```python
from build123d import *
from OCP.BRepFilletAPI import BRepFilletAPI_MakeChamfer

# Parameters (mm, degrees)
SKETCH1_R           = 2
BOSS_EXTRUDE1_DEPTH = 47
BOSS_EXTRUDE2_DEPTH = 4
FILLET1_R           = 0.2
CUT_EXTRUDE2_DEPTH  = 1
CUT_EXTRUDE2_DRAFT  = -12
CHAMFER1_SIZE       = 0.2
CHAMFER1_SIZE_2     = 0.259660706


with BuildPart() as part:
    # Sketch1 → Boss-Extrude1 (new body)
    with BuildSketch(Plane(origin=(0, 0, 0), x_dir=(1, 0, 0), z_dir=(0, 1, 0))):
        with Locations(Location((0, 0, 0), (0, 0, 270))):
            Circle(SKETCH1_R)
    extrude(amount=-BOSS_EXTRUDE1_DEPTH)

    # Sketch2 → Boss-Extrude2 (add)
    with BuildSketch(Plane(origin=(0, 0, 0), x_dir=(1, 0, 0), z_dir=(0, 1, 0))):
        Polygon((0, 5.196152423), (-4.5, 2.598076211), (-4.5, -2.598076211), (0, -5.196152423), (4.5, -2.598076211), (4.5, 2.598076211), align=None)
    extrude(amount=BOSS_EXTRUDE2_DEPTH)

    # Fillet1
    fillet1_edges = [part.edges().sort_by_distance(p)[0] for p in [
        (2.25, 0, -3.897114317),
        (4.5, 2, -2.598076211),
        (-2.25, 0, -3.897114317),
        (0, 2, -5.196152423),
        (-4.5, 0, 0),
        (-4.5, 2, -2.598076211),
        (-2.25, 0, 3.897114317),
        (-4.5, 2, 2.598076211),
        (2.25, 0, 3.897114317),
        (0, 2, 5.196152423),
        (4.5, 0, 0),
        (4.5, 2, 2.598076211),
        (2.25, 4, -3.897114317),
        (-2.25, 4, -3.897114317),
        (-4.5, 4, 0),
        (-2.25, 4, 3.897114317),
        (2.25, 4, 3.897114317),
        (4.5, 4, 0),
    ]]
    fillet(fillet1_edges, radius=FILLET1_R)


with BuildPart() as cut_extrude2_tool:
    # Sketch3 → Cut-Extrude2 (with draft: the straight prism first)
    with BuildSketch(Plane(origin=(0, 4, 0), x_dir=(1, 0, 0), z_dir=(0, 1, 0))):
        Polygon((0, 2.6), (-0.280523914, 2.5), (-0.280523914, 0.25), (-2.5, 0.25), (-2.6, 0), (-2.5, -0.25), (-0.280523914, -0.25), (-0.280523914, -2.5), (0, -2.6), (0.219476086, -2.5), (0.219476086, -0.25), (2.5, -0.25), (2.6, 0), (2.5, 0.25), (0.219476086, 0.25), (0.219476086, 2.5), align=None)
    extrude(amount=-CUT_EXTRUDE2_DEPTH)
    # Cut-Extrude2: the draft: its side faces are tilted about the plane it starts from
    cut_extrude2_sides = [cut_extrude2_tool.faces().sort_by_distance(p)[0] for p in [
        (-0.140261957, 3.5, -2.55),
        (-0.280523914, 3.5, -1.375),
        (-1.390261957, 3.5, -0.25),
        (-2.55, 3.5, -0.125),
        (-2.55, 3.5, 0.125),
        (-1.390261957, 3.5, 0.25),
        (-0.280523914, 3.5, 1.375),
        (-0.140261957, 3.5, 2.55),
        (0.109738043, 3.5, 2.55),
        (0.219476086, 3.5, 1.375),
        (1.359738043, 3.5, 0.25),
        (2.55, 3.5, 0.125),
        (2.55, 3.5, -0.125),
        (1.359738043, 3.5, -0.25),
        (0.219476086, 3.5, -1.375),
        (0.109738043, 3.5, -2.55),
    ]]
    draft(cut_extrude2_sides, Plane(origin=(0, 4, 0), x_dir=(1, 0, 0), z_dir=(0, 1, 0)), CUT_EXTRUDE2_DRAFT)


with BuildPart() as part_1:
    add(part.part)

    # Cut-Extrude2: cut by cut_extrude2_tool
    add(cut_extrude2_tool.part, mode=Mode.SUBTRACT)

    # Chamfer1
    chamfer1_edges_1 = [part_1.edges().sort_by_distance(p)[0] for p in [
        (0.109738043, 4, -2.55),
    ]]
    chamfer1_side_1 = [part_1.faces().sort_by_distance(p)[0] for p in [
        (0.111396527, 4, -2.553639977),
    ]]
    chamfer1_edges_2 = [part_1.edges().sort_by_distance(p)[0] for p in [
        (-0.140261957, 4, -2.55),
    ]]
    chamfer1_side_2 = [part_1.faces().sort_by_distance(p)[0] for p in [
        (-0.141605074, 4, -2.553767763),
    ]]
    chamfer1_edges_3 = [part_1.edges().sort_by_distance(p)[0] for p in [
        (-0.280523914, 4, -1.375),
    ]]
    chamfer1_side_3 = [part_1.faces().sort_by_distance(p)[0] for p in [
        (-0.284523914, 4, -1.375),
    ]]
    chamfer1_edges_4 = [part_1.edges().sort_by_distance(p)[0] for p in [
        (-1.390261957, 4, -0.25),
    ]]
    chamfer1_side_4 = [part_1.faces().sort_by_distance(p)[0] for p in [
        (-1.390261957, 4, -0.254),
    ]]
    chamfer1_edges_5 = [part_1.edges().sort_by_distance(p)[0] for p in [
        (-2.55, 4, -0.125),
    ]]
    chamfer1_side_5 = [part_1.faces().sort_by_distance(p)[0] for p in [
        (-2.553713907, 4, -0.126485563),
    ]]
    chamfer1_edges_6 = [part_1.edges().sort_by_distance(p)[0] for p in [
        (-2.55, 4, 0.125),
    ]]
    chamfer1_side_6 = [part_1.faces().sort_by_distance(p)[0] for p in [
        (-2.553713907, 4, 0.126485563),
    ]]
    chamfer1_edges_7 = [part_1.edges().sort_by_distance(p)[0] for p in [
        (-1.390261957, 4, 0.25),
    ]]
    chamfer1_side_7 = [part_1.faces().sort_by_distance(p)[0] for p in [
        (-1.390261957, 4, 0.254),
    ]]
    chamfer1_edges_8 = [part_1.edges().sort_by_distance(p)[0] for p in [
        (-0.280523914, 4, 1.375),
    ]]
    chamfer1_side_8 = [part_1.faces().sort_by_distance(p)[0] for p in [
        (-0.284523914, 4, 1.375),
    ]]
    chamfer1_edges_9 = [part_1.edges().sort_by_distance(p)[0] for p in [
        (-0.140261957, 4, 2.55),
    ]]
    chamfer1_side_9 = [part_1.faces().sort_by_distance(p)[0] for p in [
        (-0.141605074, 4, 2.553767763),
    ]]
    chamfer1_edges_10 = [part_1.edges().sort_by_distance(p)[0] for p in [
        (0.109738043, 4, 2.55),
    ]]
    chamfer1_side_10 = [part_1.faces().sort_by_distance(p)[0] for p in [
        (0.111396527, 4, 2.553639977),
    ]]
    chamfer1_edges_11 = [part_1.edges().sort_by_distance(p)[0] for p in [
        (0.219476086, 4, 1.375),
    ]]
    chamfer1_side_11 = [part_1.faces().sort_by_distance(p)[0] for p in [
        (0.223476086, 4, 1.375),
    ]]
    chamfer1_edges_12 = [part_1.edges().sort_by_distance(p)[0] for p in [
        (1.359738043, 4, 0.25),
    ]]
    chamfer1_side_12 = [part_1.faces().sort_by_distance(p)[0] for p in [
        (1.359738043, 4, 0.254),
    ]]
    chamfer1_edges_13 = [part_1.edges().sort_by_distance(p)[0] for p in [
        (2.55, 4, 0.125),
    ]]
    chamfer1_side_13 = [part_1.faces().sort_by_distance(p)[0] for p in [
        (2.553713907, 4, 0.126485563),
    ]]
    chamfer1_edges_14 = [part_1.edges().sort_by_distance(p)[0] for p in [
        (2.55, 4, -0.125),
    ]]
    chamfer1_side_14 = [part_1.faces().sort_by_distance(p)[0] for p in [
        (2.553713907, 4, -0.126485563),
    ]]
    chamfer1_edges_15 = [part_1.edges().sort_by_distance(p)[0] for p in [
        (1.359738043, 4, -0.25),
    ]]
    chamfer1_side_15 = [part_1.faces().sort_by_distance(p)[0] for p in [
        (1.359738043, 4, -0.254),
    ]]
    chamfer1_edges_16 = [part_1.edges().sort_by_distance(p)[0] for p in [
        (0.219476086, 4, -1.375),
    ]]
    chamfer1_side_16 = [part_1.faces().sort_by_distance(p)[0] for p in [
        (0.223476086, 4, -1.375),
    ]]
    chamfer1 = BRepFilletAPI_MakeChamfer(part_1.part.solid().wrapped)
    for e in chamfer1_edges_1:
        chamfer1.Add(CHAMFER1_SIZE - 0.0001, CHAMFER1_SIZE_2 - 0.0001, e.wrapped, chamfer1_side_1[0].wrapped)
    for e in chamfer1_edges_2:
        chamfer1.Add(CHAMFER1_SIZE - 0.0001, CHAMFER1_SIZE_2 - 0.0001, e.wrapped, chamfer1_side_2[0].wrapped)
    for e in chamfer1_edges_3:
        chamfer1.Add(CHAMFER1_SIZE - 0.0001, CHAMFER1_SIZE_2 - 0.0001, e.wrapped, chamfer1_side_3[0].wrapped)
    for e in chamfer1_edges_4:
        chamfer1.Add(CHAMFER1_SIZE - 0.0001, CHAMFER1_SIZE_2 - 0.0001, e.wrapped, chamfer1_side_4[0].wrapped)
    for e in chamfer1_edges_5:
        chamfer1.Add(CHAMFER1_SIZE - 0.0001, CHAMFER1_SIZE_2 - 0.0001, e.wrapped, chamfer1_side_5[0].wrapped)
    for e in chamfer1_edges_6:
        chamfer1.Add(CHAMFER1_SIZE - 0.0001, CHAMFER1_SIZE_2 - 0.0001, e.wrapped, chamfer1_side_6[0].wrapped)
    for e in chamfer1_edges_7:
        chamfer1.Add(CHAMFER1_SIZE - 0.0001, CHAMFER1_SIZE_2 - 0.0001, e.wrapped, chamfer1_side_7[0].wrapped)
    for e in chamfer1_edges_8:
        chamfer1.Add(CHAMFER1_SIZE - 0.0001, CHAMFER1_SIZE_2 - 0.0001, e.wrapped, chamfer1_side_8[0].wrapped)
    for e in chamfer1_edges_9:
        chamfer1.Add(CHAMFER1_SIZE - 0.0001, CHAMFER1_SIZE_2 - 0.0001, e.wrapped, chamfer1_side_9[0].wrapped)
    for e in chamfer1_edges_10:
        chamfer1.Add(CHAMFER1_SIZE - 0.0001, CHAMFER1_SIZE_2 - 0.0001, e.wrapped, chamfer1_side_10[0].wrapped)
    for e in chamfer1_edges_11:
        chamfer1.Add(CHAMFER1_SIZE - 0.0001, CHAMFER1_SIZE_2 - 0.0001, e.wrapped, chamfer1_side_11[0].wrapped)
    for e in chamfer1_edges_12:
        chamfer1.Add(CHAMFER1_SIZE - 0.0001, CHAMFER1_SIZE_2 - 0.0001, e.wrapped, chamfer1_side_12[0].wrapped)
    for e in chamfer1_edges_13:
        chamfer1.Add(CHAMFER1_SIZE - 0.0001, CHAMFER1_SIZE_2 - 0.0001, e.wrapped, chamfer1_side_13[0].wrapped)
    for e in chamfer1_edges_14:
        chamfer1.Add(CHAMFER1_SIZE - 0.0001, CHAMFER1_SIZE_2 - 0.0001, e.wrapped, chamfer1_side_14[0].wrapped)
    for e in chamfer1_edges_15:
        chamfer1.Add(CHAMFER1_SIZE - 0.0001, CHAMFER1_SIZE_2 - 0.0001, e.wrapped, chamfer1_side_15[0].wrapped)
    for e in chamfer1_edges_16:
        chamfer1.Add(CHAMFER1_SIZE - 0.0001, CHAMFER1_SIZE_2 - 0.0001, e.wrapped, chamfer1_side_16[0].wrapped)
    add(Compound.cast(chamfer1.Shape()), mode=Mode.REPLACE)  # a hair under: the kernel refuses the full size


solid = part_1.part
```
Source: CAD feature listing. Evaluate the final solid. Frame: model axes, mm. A direction names the side the tool comes from. Round coordinates to 2 decimals unless told otherwise and drop trailing zeros. Loops run counter-clockwise (first coordinate to the right, second up) from the corner with the lowest first, then second, coordinate; pieces in that order, holes last. Notation, with made-up numbers: M -8.75,32.25 L 44.25,32.25 A24 cw 44.25,45.25 Z; hole C 63,84 d4. An arc over 180 degrees is marked long. Put each result on its own line as item: value.
(1) Section A-A, the plane y = -32.5. Return loops of the section in (x, z), and give its area (3 significant figures).
Solutions:
outline: C 0,0 d4
area: 12.6 mm²
(2) First-contact query: pin 1 (1.5 mm diameter, centred on y = -34.5, z = 4, fed in from +X); pin 2 (5 mm diameter, centred on x = 0.5, y = -35, fed in from -Z). Flat tips, straight axial feed; report the tip coordinate or a pass-through.
Solutions:
pin 1: through
pin 2: z = -2
(3) Access query for faces 1 (the face through (-2, 0, 1)), 2 (the face through (2.22, 1.975, 3.914)). Directions: +Z, -Z, +X, -X, +Y, -Y. A direction counts if a zero-diameter tool reaches every point of the face in a straight line with its end or side. Return the directions, or none.
Solutions:
face 1: -Y
face 2: +Z, +X, +Y, -Y
(4) Pull-direction query (Z, two-part tool) for faces 3 (the face through (-2.19, 3.943, 3.862)), 4 (the face through (0, -47, 0)), 5 (the face through (-2.25, 3.94, -3.83)); classes: released by +Z, released by -Z, zero draft, split by the parting line, or undercut.
Solutions:
face 3: released by +Z
face 4: zero draft
face 5: released by -Z
(5) Ray query, line 1 (Y direction, x = 0, z = -3.5); line 2 (X direction, y = -23.5, z = 1.5); line 3 (Z direction, x = -0.25, y = -16). Return the intervals inside material, ascending. Write a range as [from, to].
Solutions:
line 1: [0, 4]
line 2: [-1.32, 1.32]
line 3: [-1.98, 1.98]
